Part model, mm, in its own coordinate system. Face numbers are marked on the shaded views. A direction names the side the tool comes from. Give positions to 0.01 mm unless a question says otherwise; leave off trailing zeros. Order: outer loops, then holes, each group sorted by start corner. A loop starts at its lowest first (then second) coordinate and runs counter-clockwise, first axis right, second up.
1. Slice it at B-B on y = -34. List the corners of the cut face in (x, z), and give its area (3 significant figures).
2. Which spindle directions (+Z, -Z, +X, -X, +Y, -Y) get a long thin tool onto all of the face, cutting with end or side? Do the marked faces 4 and 5. Say none if no direction does.
3. Mould opens along X. For the marked faces 1, 2 and 3 say: +X half, -X half, draft (parallel to the pull), parting line (faces both ways), or undercut.
4. Slice it at A-A on x = 8. List the corners of the cut face in (y, z), and give its area (3 significant figures).
5. Drop flat-ended pins along their axis: pin 1 Ø5.5 at (y, z) = (32, 5.5) entering from -X; pin 2 Ø6 at (x, z) = (-9, 8) entering from -Y; pin 3 Ø1.5 at (x, z) = (-3, 16) entering from -Y. Give the stop position or say it passes through.
6. Probe line 1 (X direction, y = -10, z = 9.5); line 2 (X direction, y = 22.5, z = 1.5); line 3 (Z direction, x = 4.5, y = -11.5). List the from-to ranges inside material, lowest first.
from build123d import *

# Parameters (mm, degrees)
F1_DEPTH = 18
F3_DEPTH = 10


with BuildPart() as f1:
    # F0 (on Top) → F1 (new body)
    with BuildSketch(Plane.XY):
        with BuildLine():
            add(Edge.make_bspline(
                [(9.5007545576, 39), (12.4635481183, 34.8866982316), (20.8197259912, 23.2484041941), (14.2138642453, -9.70977485), (9.7924165598, -31.0301836975)],
                knots=[0, 0, 0, 0, 0.3533498834, 1, 1, 1, 1], degree=3))
            Line((9.5007545576, 39), (6.5015091152, 39))
            Line((6.5015091152, 39), (6.5015091152, 14))
            ThreePointArc((6.5015091152, 14), (3.4015161475, 12.5111942523), (0.0007545576, 12))
            ThreePointArc((0.0007545576, 12), (-3.4000070322, 12.5111942523), (-6.5, 14))
            Line((-6.5, 14), (-6.5, 39))
            Line((-6.5, 39), (-9.4992454424, 39))
            add(Edge.make_bspline(
                [(-9.4992454424, 39), (-12.4620390031, 34.8866982316), (-20.818216876, 23.2484041941), (-14.2123551301, -9.70977485), (-9.7909074446, -31.0301836975)],
                knots=[0, 0, 0, 0, 0.3533498834, 1, 1, 1, 1], degree=3))
            ThreePointArc((-9.7909074446, -31.0301836975), (0.0007545576, -38.9995790498), (9.7924165598, -31.0301836975))
        make_face()
    extrude(amount=F1_DEPTH)

    # F2 (on face) → F3 (cut)
    with BuildSketch(Plane.XY.offset(18)):
        with BuildLine():
            ThreePointArc((0.0007545576, -1), (-2.83164725, -1.5166352097), (-5.2992454424, -3))
            Line((-5.2992454424, -3), (-5.2992454424, -23.3))
            ThreePointArc((-5.2992454424, -23.3), (-2.8320002359, -24.7832316067), (0, -25.3))
            ThreePointArc((0, -25.3), (0.0007545576, -25.3000000355), (0.0015091152, -25.3))
            ThreePointArc((0.0015091152, -25.3), (2.8335093511, -24.7832316067), (5.3007545576, -23.3))
            Line((5.3007545576, -23.3), (5.3007545576, -3))
            ThreePointArc((5.3007545576, -3), (2.8331563653, -1.5166352097), (0.0007545576, -1))
        make_face()
    extrude(amount=-F3_DEPTH, mode=Mode.SUBTRACT)


solid = f1.part
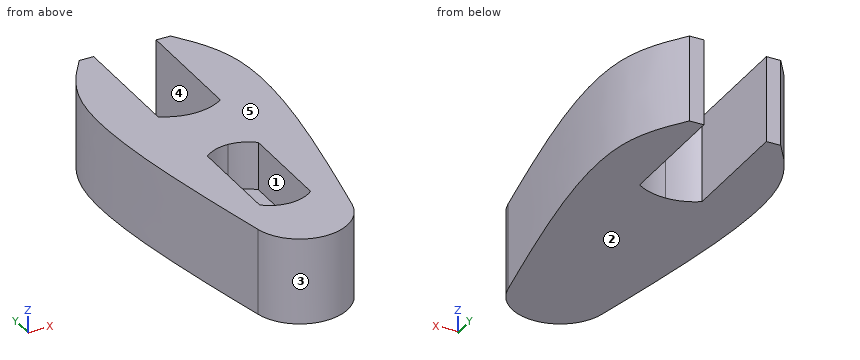
Data:
1. outline: (-8.66, 0) - (8.66, 0) - (8.66, 18) - (-8.66, 18) - close
1. area: 312 mm2
2. face 4: +Z, -Z, +Y
2. face 5: +Z, +X, -X, +Y, -Y
3. face 1: undercut
3. face 2: draft
3. face 3: parting line
4. outline: (-35, 0) - (39, 0) - (39, 18) - (-35, 18) - close
4. area: 1,330 mm2
5. pin 1: stops at x = -15.14
5. pin 2: stops at y = -37
5. pin 3: stops at y = -38.74
6. line 1: x = -13.94 to -5.3, 5.3 to 13.95
6. line 2: x = -16.7 to -6.5, 6.5 to 16.71
6. line 3: z = 0 to 8
